Source: CAD feature listing. Evaluate the final solid. Frame: model axes, mm. Coordinates: 2 decimals unless noted, no trailing zeros. Loops run counter-clockwise (first coordinate to the right, second up) from the corner with the lowest first, then second, coordinate; pieces in that order, holes last.
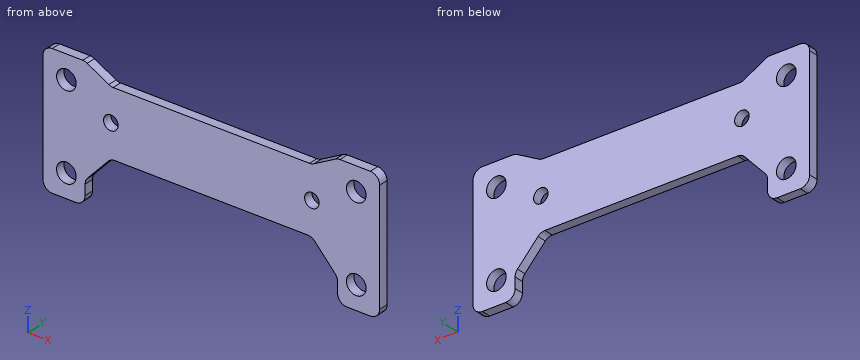
```python
from build123d import *

# Parameters (mm, degrees)
SKETCH1_R           = 2.1
SKETCH1_R_2         = 1.55
BOSS_EXTRUDE1_DEPTH = 2
FILLET1_R           = 2


with BuildPart() as part:
    # Sketch1 → Boss-Extrude1 (new body)
    with BuildSketch(Plane(origin=(0, 0, 0), x_dir=(1, 0, 0), z_dir=(0, 1, 0))):
        Polygon((-67, -5), (-58, -5), (-52.5, -2), (-9.5, -2), (-4, -5), (5, -5), (5, 23), (-4, 23), (-4, 18), (-9.5, 12), (-52.5, 12), (-58, 18), (-58, 23), (-67, 23), align=None)
        Circle(SKETCH1_R, mode=Mode.SUBTRACT)
        with Locations((0, 18)):
            Circle(SKETCH1_R, mode=Mode.SUBTRACT)
        with Locations((-62, 18)):
            Circle(SKETCH1_R, mode=Mode.SUBTRACT)
        with Locations((-62, 0)):
            Circle(SKETCH1_R, mode=Mode.SUBTRACT)
        with Locations((-9.5, 5)):
            Circle(SKETCH1_R_2, mode=Mode.SUBTRACT)
        with Locations((-52.5, 5)):
            Circle(SKETCH1_R_2, mode=Mode.SUBTRACT)
    extrude(amount=BOSS_EXTRUDE1_DEPTH)

    # Fillet1
    fillet1_edges = [part.edges().sort_by_distance(p)[0] for p in [
        (-4, 1, 5),
        (-9.5, 1, 2),
        (-52.5, 1, 2),
        (-58, 1, 5),
        (-67, 1, 5),
        (-67, 1, -23),
        (-58, 1, -23),
        (-58, 1, -18),
        (-52.5, 1, -12),
        (-9.5, 1, -12),
        (-4, 1, -18),
        (-4, 1, -23),
        (5, 1, -23),
        (5, 1, 5),
    ]]
    fillet(fillet1_edges, radius=FILLET1_R)


solid = part.part
```
Q1. Section query C-C on y = 0.6. Count the separate pieces of the cut face and the enclosed holes in it, then the cut area to 3 significant figures.
Q2. Material intervals for line 1 along Z through (x, y) = (0, 1.6); line 2 along X through (y, z) = (1.05, 0); line 3 along X through (y, z) = (0.55, -5), sorted ascending.
Q3. Section query B-B on z = -5. Return the cut outline in (x, y).
Q4. First-contact query: pin 1 Ø1 at (x, y) = (-30.5, 1.5) entering from +Z; pin 2 Ø0.6 at (x, y) = (-25, 1.5) entering from -Z. Flat tips, straight axial feed; report the tip coordinate or a pass-through.
Q5. Section query A-A on x = -62. Return the cut outline in (y, z).
Q6. Section query D-D on z = -14. Return the cut outline in (x, y).
Resolved:
1. separate pieces: 1
1. enclosed holes: 6
1. area: 1,230 mm2
2. line 1: z = -23 to -20.1, -15.9 to -2.1, 2.1 to 5
2. line 2: x = -67 to -64.1, -59.9 to -2.1, 2.1 to 5
2. line 3: x = -67 to -54.05, -50.95 to -11.05, -7.95 to 5
3. outline: (-67, 0) - (-54.05, 0) - (-54.05, 2) - (-67, 2) - close; (-50.95, 0) - (-11.05, 0) - (-11.05, 2) - (-50.95, 2) - close; (-7.95, 0) - (5, 0) - (5, 2) - (-7.95, 2) - close
4. pin 1: stops at z = 2
4. pin 2: stops at z = -12
5. outline: (0, -23) - (2, -23) - (2, -20.1) - (0, -20.1) - close; (0, -15.9) - (2, -15.9) - (2, -2.1) - (0, -2.1) - close; (0, 2.1) - (2, 2.1) - (2, 5) - (0, 5) - close
6. outline: (-67, 0) - (-54.33, 0) - (-54.33, 2) - (-67, 2) - close; (-7.67, 0) - (5, 0) - (5, 2) - (-7.67, 2) - close
